The model under review builds one solid part; all positions refer to its coordinate system, in mm. A direction names the side the tool comes from. Round coordinates to 2 decimals unless told otherwise and drop trailing zeros. Order: outer loops, then holes, each group sorted by start corner. A loop starts at its lowest first (then second) coordinate and runs counter-clockwise, first axis right, second up.
1) Consider section B-B (z = -43). Give the boundary of the cut face in (x, y), then the cut area to 3 significant figures.
2) Clearance check with flat-ended pins moving along their axes: P1, Ø6, axis at y = 6.5, z = 33, coming from the +X side; P2, Ø8, axis at x = -33.5, y = 8, coming from the +Z side; P3, Ø6.5, axis at x = 57.5, y = 6.5, coming from the -Z side. State where each tip first meets the part, or that it passes through.
3) Consider section C-C (y = 7). Give the number of separate pieces and of enclosed holes in the cut face, then the cut area to 3 significant figures.
4) Machinability: for faces 1 (the face through (59.1, 10.14, 59.14)), 2 (the face through (56, 10, 38)), which of the approach directions +Z, -Z, +X, -X, +Y, -Y give a long, thin tool a straight path to every point of the face, cutting with its end or side? Answer none if there is none.
5) To check wall thickness, follow L1, parallel to Z at x = -9, y = 2.4; L2, parallel to X at y = 18, z = 1. State the ranges of each line that lie inside material, in increasing order.
6) Consider section A-A (x = 25). Give the boundary of the cut face in (y, z).
7) Mouldability with a two-part tool opening along Z and no side actions: class faces 3 (the face through (-8.703, 7.395, -15.75)), 4 (the face through (-36.3, 7.4, -43.9)), 5 (the face through (-60, 10, -8)), 6 (the face through (-10, 10, -60)) as pulls with the +Z half, pulls with the -Z half, needs draft (parallel to the pull), parting line crosses it, or undercut.
from build123d import *

# Parameters (mm, degrees)
SCHIZZO1_W                   = 120
SCHIZZO1_H                   = 120
ESTRUSIONE_ESTRUSIONE1_DEPTH = 20
SCHIZZO5_R                   = 5
TAGLIO_ESTRUSIONE2_DEPTH     = 87.168439698
RIPETIZIONE_A_L1_COUNT       = 3
RIPETIZIONE_A_L1_PITCH       = 34
RIPETIZIONE_A_L1_COUNT_DIR2  = 3
RIPETIZIONE_A_L1_PITCH_DIR2  = 34
SCHIZZO7_W                   = 98
SCHIZZO7_H                   = 18
SCHIZZO7_W_2                 = 18
SCHIZZO7_H_2                 = 98
TAGLIO_ESTRUSIONE3_DEPTH     = 20
SMUSSO1_SIZE                 = 10
SCHIZZO8_R                   = 6.5
TAGLIO_ESTRUSIONE4_DEPTH     = 20
RIPETIZIONE_A_L2_COUNT       = 2
RIPETIZIONE_A_L2_PITCH       = 34
RIPETIZIONE_A_L2_COUNT_DIR2  = 2
RIPETIZIONE_A_L2_PITCH_DIR2  = 32
RACCORDO1_R                  = 3


with BuildPart() as part:
    # Schizzo1 → Estrusione-Estrusione1 (new body)
    with BuildSketch(Plane(origin=(0, 0, 0), x_dir=(1, 0, 0), z_dir=(0, 1, 0))):
        Rectangle(SCHIZZO1_W, SCHIZZO1_H)
    extrude(amount=ESTRUSIONE_ESTRUSIONE1_DEPTH)

    # Schizzo6 → Taglia-Rivoluzione4 (revolve, cut)
    with BuildSketch(Plane.ZY.offset(43)):
        Polygon((-43, 20), (-27, 20), (-38, 5), (-43, 5), align=None)
    taglia_rivoluzione4 = revolve(axis=Axis((-43, 5, -43), (0, 1, 0)), mode=Mode.SUBTRACT)

    # Schizzo5 → Taglio-Estrusione2 (cut, symmetric)
    with BuildSketch(Plane(origin=(0, 5, 0), x_dir=(-1, 0, 0), z_dir=(0, -1, 0))):
        with Locations(Location((43, 43, 0), (0, 0, 90))):
            Circle(SCHIZZO5_R)
    taglio_estrusione2 = extrude(amount=TAGLIO_ESTRUSIONE2_DEPTH, both=True, mode=Mode.SUBTRACT)

    # Ripetizione a L1: Taglia-Rivoluzione4, Taglio-Estrusione2 3 × 3
    with Locations(*[(i * RIPETIZIONE_A_L1_PITCH, 0, j * RIPETIZIONE_A_L1_PITCH_DIR2) for i in range(RIPETIZIONE_A_L1_COUNT) for j in range(RIPETIZIONE_A_L1_COUNT_DIR2) if (i, j) != (0, 0)]):
        add(taglia_rivoluzione4, mode=Mode.SUBTRACT)
        add(taglio_estrusione2, mode=Mode.SUBTRACT)

    # Schizzo7 → Taglio-Estrusione3 (cut)
    with BuildSketch(Plane(origin=(0, 20, 0), x_dir=(1, 0, 0), z_dir=(0, 1, 0))):
        with Locations((-11, -51)):
            Rectangle(SCHIZZO7_W, SCHIZZO7_H)
        with Locations((51, 11)):
            Rectangle(SCHIZZO7_W_2, SCHIZZO7_H_2)
    extrude(amount=-TAGLIO_ESTRUSIONE3_DEPTH, mode=Mode.SUBTRACT)

    # Smusso1
    smusso1_edges = [part.edges().sort_by_distance(p)[0] for p in [
        (-60, 10, -60),
        (38, 10, 42),
        (-60, 10, 42),
        (42, 10, 38),
        (42, 10, -60),
    ]]
    chamfer(smusso1_edges, length=SMUSSO1_SIZE)

    # Schizzo8 → Taglio-Estrusione4 (cut)
    with BuildSketch(Plane(origin=(0, 20, 0), x_dir=(1, 0, 0), z_dir=(0, 1, 0))):
        with Locations(Location((8, -8, 0), (0, 0, 270))):
            Circle(SCHIZZO8_R)
    taglio_estrusione4 = extrude(amount=-TAGLIO_ESTRUSIONE4_DEPTH, mode=Mode.SUBTRACT)

    # Ripetizione a L2: Taglio-Estrusione4 2 × 2
    with Locations(*[(-j * RIPETIZIONE_A_L2_PITCH_DIR2, 0, -i * RIPETIZIONE_A_L2_PITCH) for i in range(RIPETIZIONE_A_L2_COUNT) for j in range(RIPETIZIONE_A_L2_COUNT_DIR2) if (i, j) != (0, 0)]):
        add(taglio_estrusione4, mode=Mode.SUBTRACT)

    # Raccordo1
    raccordo1_edges = [part.edges().sort_by_distance(p)[0] for p in [
        (60, 10, 60),
    ]]
    fillet(raccordo1_edges, radius=RACCORDO1_R)


solid = part.part
Answer below:
1. outline: (-60, 0) - (-48, 0) - (-48, 5) - (-59, 20) - (-60, 20) - close; (-38, 0) - (-14, 0) - (-14, 5) - (-25, 20) - (-27, 20) - (-38, 5) - close; (-4, 0) - (20, 0) - (20, 5) - (9, 20) - (7, 20) - (-4, 5) - close; (30, 0) - (42, 0) - (42, 20) - (41, 20) - (30, 5) - close
1. area: 945 mm2
2. P1: stops at x = 50
2. P2: stops at z = 42
2. P3: stops at z = 38
3. separate pieces: 1
3. enclosed holes: 13
3. area: 9,110 mm2
4. face 1: +Z, +X, +Y, -Y
4. face 2: -Z, +X, +Y, -Y
5. L1: z = -60 to -48, -38 to -14, -4 to 20, 30 to 42
5. L2: x = -60 to -53.55, -32.45 to -19.55, 1.55 to 14.45, 35.55 to 42
6. outline: (0, -60) - (20, -60) - (20, -59) - (5, -48) - (0, -48) - close; (0, -38) - (5, -38) - (20, -27) - (20, -25) - (5, -14) - (0, -14) - close; (0, -4) - (5, -4) - (20, 7) - (20, 9) - (5, 20) - (0, 20) - close; (0, 30) - (5, 30) - (20, 41) - (20, 42) - (0, 42) - close
7. face 3: undercut
7. face 4: undercut
7. face 5: needs draft
7. face 6: pulls with the -Z half
